Could you check a few things on this drawing? It's one solid part, dimensions in mm from its lowest x, y, z. Round coordinates to 2 decimals unless told otherwise and drop trailing zeros. Loops run counter-clockwise (first coordinate to the right, second up) from the corner with the lowest first, then second, coordinate; pieces in that order, holes last. Notation, with made-up numbers: M 46,64.25 L 59,64.25 A14 ccw 59,70.25 Z; hole C 75,5.5 d8. An arc over 180 degrees is marked long. Use a Markdown table: item, result. Add a question column.
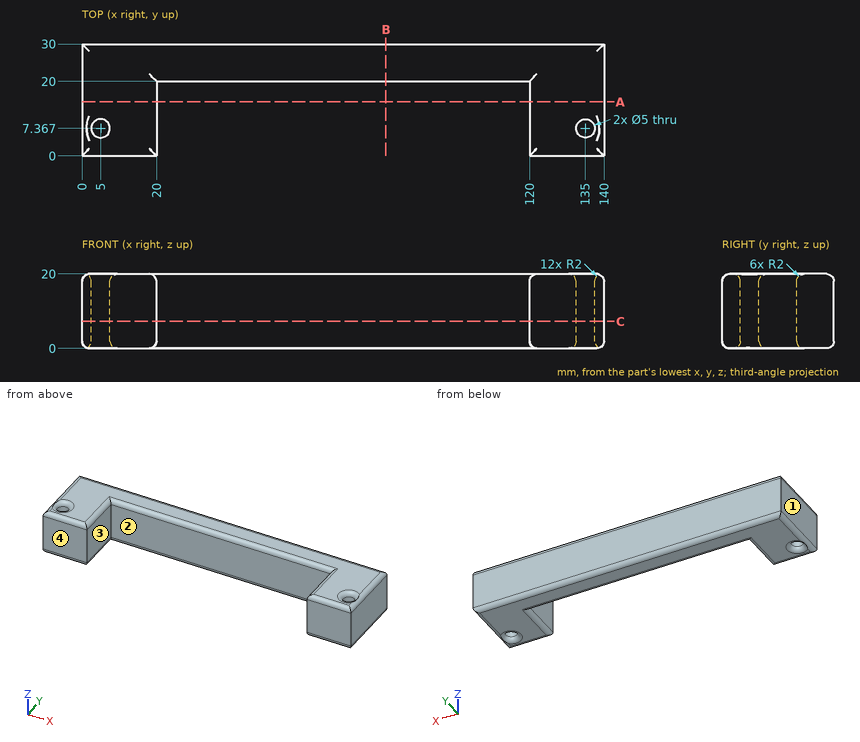
(1) If I drill on probe 1 along Y at (x, z) = (135, 6.5); probe 2 along X at (y, z) = (14, 18.25); probe 3 along X at (y, z) = (9, 7.25), over which ranges is the centre line in solid material (lowest first)? Write a range as [from, to].
(2) Thinking about a two-plate mould opening in X: for the marked faces 1, 2, 3 and 4, which applies, released by +X, released by -X, zero draft, split by the parting line, or undercut?
(3) Suppose I cut it at B-B on x = 81.5. List the corners of the cut face in (y, z) for me.
(4) Suppose I cut it at A-A on y = 14.5. List the corners of the cut face in (x, z) for me.
(5) I'm going to push a flat-ended pin straight in: pin 1 (4.5 mm diameter, centred on x = 135, y = 7.37, fed in from +Z). Where does the tip first touch, or does it pass through?
(6) Suppose I cut it at C-C on z = 7.25. List the corners of the cut face in (x, y) for me, and give its area (3 significant figures).
Results below:
| question | item | result |
|---|---|---|
| 1 | probe 1 | y = [0, 4.87], [9.87, 30] |
| 1 | probe 2 | x = [0.02, 19.98], [120.02, 139.98] |
| 1 | probe 3 | x = [0, 3.11], [6.89, 20], [120, 133.11], [136.89, 140] |
| 2 | face 1 | released by -X |
| 2 | face 2 | undercut |
| 2 | face 3 | undercut |
| 2 | face 4 | zero draft |
| 3 | outline | M 20,2 A2 ccw 22,0 L 28,0 A2 ccw 30,2 L 30,18 A2 ccw 28,20 L 22,20 A2 ccw 20,18 Z |
| 4 | outline | M 0,2 A2 ccw 2,0 L 18,0 A2 ccw 20,2 L 20,18 A2 ccw 18,20 L 2,20 A2 ccw 0,18 Z; M 120,2 A2 ccw 122,0 L 138,0 A2 ccw 140,2 L 140,18 A2 ccw 138,20 L 122,20 A2 ccw 120,18 Z |
| 5 | pin 1 | passes through |
| 6 | outline | M 0,0 L 20,0 L 20,20 L 120,20 L 120,0 L 140,0 L 140,30 L 0,30 Z; hole C 5,7.37 d5; hole C 135,7.37 d5 |
| 6 | area | 2,160 mm² |
